from build123d import *

# Parameters (mm, degrees)
F1_DEPTH = 250
F3_DEPTH = 160
F4_T     = -2


with BuildPart() as f1:
    # F0 (on Front) → F1 (new body)
    with BuildSketch(Plane.XZ):
        Polygon((72.809999, 73.434824), (-47.190001, 73.434824), (-47.190001, -46.565176), (72.809999, -46.565176), (112.809999, -46.565176), (112.809999, 73.434824), align=None)
    extrude(amount=F1_DEPTH)

    # F2 (on face) → F3 (cut, through all)
    with BuildSketch(Plane.YZ.offset(112.809999)):
        Polygon((-250, 73.434824), (-250, 7.656341), (-226.05859, 73.434824), align=None)
    extrude(amount=-F3_DEPTH, mode=Mode.SUBTRACT)

    # F4
    f4_openings = [f1.faces().sort_by_distance(p)[0] for p in [
        (32.809999, -113.029295, 73.434824),
    ]]
    offset(amount=F4_T, openings=f4_openings)


solid = f1.part
Input: part model. Units: mm. Frame: model coordinates. A direction names the side the tool comes from. Coordinates: 2 decimals unless noted, no trailing zeros. Write each loop counter-clockwise with the first axis right and the second up, starting at its lowest first coordinate (ties: lowest second). Pieces come first, ordered by that corner, then holes. Notation, with made-up numbers: M 27,22 L 46,22 A7 ccw 46,35 Z; hole C 4,71.25 d2. An arc over 180 degrees is marked long. Answer as a JSON object with one key per item and string values. Group by question number.
(1) Set-up query: faces 4 (the face through (32, -248, -18)), 5 (the face through (32, -123, -46.565)), 6 (the face through (32, -2, 15)). Return all of +Z, -Z, +X, -X, +Y, -Y with unobstructed straight access to the full face (end or side cutting, diameter ignored); none if empty.
(2) Section D-D on z = 46. Output: boundary loops of the cut face in (x, y), plus the area to 3 significant figures.
(3) Ray query, line 1 along X through (y, z) = (-189, 59); line 2 along Y through (x, z) = (85, -5.5); line 3 along Z through (x, y) = (100.5, -117). Return the intervals inside material, ascending. Write a range as [from, to].
(4) Section A-A on x = -14. Output: boundary loops of the cut face in (y, z), plus the area to 3 significant figures.
(5) Mould query, pull axis Y, two halves, no side actions, for faces 1 (the face through (33.902, -236.134, 39.906)), 2 (the face through (-47.19, -123, 14)), 3 (the face through (32, 0, 14)). Classes: pulls with the +Y half, pulls with the -Y half, needs draft (parallel to the pull), parting line crosses it, or undercut.
(6) Section C-C on y = -218.5. Output: boundary loops of the cut face in (x, z).
(7) Section B-B on z = -34.5. Output: boundary loops of the cut face in (x, y).
(8) Contact query for flat-ended pins moving along their axis: P1, Ø2, axis at x = -0.5, z = 3, coming from the +Y side; P2, Ø12, axis at x = 90.5, y = -120.5, coming from the +Z side; P3, Ø12, axis at x = 35.5, z = 23.5, coming from the -Y side. Output: stop coordinate, or through.
Result set:
{
 "1": {"face 4": "none", "face 5": "-Z, +X, -X, +Y, -Y", "face 6": "+Z"},
 "2": {"outline": "M -47.19,-236.04 L 112.81,-236.04 L 112.81,0 L -47.19,0 Z; hole M -45.19,-233.92 L 110.81,-233.92 L 110.81,-2 L -45.19,-2 Z", "area": "1,590 mm2"},
 "3": {"line 1": "x = [-47.19, -45.19], [110.81, 112.81]", "line 2": "y = [-250, -248], [-2, 0]", "line 3": "z = [-46.57, -44.57]"},
 "4": {"outline": "M -250,-46.57 L 0,-46.57 L 0,73.43 L -2,73.43 L -2,-44.57 L -248,-44.57 L -248,7.3 L -223.93,73.43 L -226.06,73.43 L -250,7.66 Z", "area": "980 mm2"},
 "5": {"face 1": "undercut", "face 2": "needs draft", "face 3": "pulls with the +Y half"},
 "6": {"outline": "M -47.19,-46.57 L 112.81,-46.57 L 112.81,73.43 L 110.81,73.43 L 110.81,-44.57 L -45.19,-44.57 L -45.19,73.43 L -47.19,73.43 Z"},
 "7": {"outline": "M -47.19,-250 L 112.81,-250 L 112.81,0 L -47.19,0 Z; hole M -45.19,-248 L 110.81,-248 L 110.81,-2 L -45.19,-2 Z"},
 "8": {"P1": "stops at y = 0", "P2": "stops at z = -44.57", "P3": "stops at y = -246.42"}
}
